The listing builds one solid part. Answer for the finished solid, in the listing's coordinates (mm). A direction names the side the tool comes from. Give positions to 0.01 mm unless a question says otherwise; leave off trailing zeros. Write each loop counter-clockwise with the first axis right and the second up, starting at its lowest first coordinate (ties: lowest second). Pieces come first, ordered by that corner, then holes. Notation, with made-up numbers: (51, 26.25) - (108, 26.25) arc R17 ccw to (108, 48.25) - close; hole circle Ø10 at (-39, 69.25). An arc over 180 degrees is marked (long way). Return JSON: item names as keys, results as strings.
from build123d import *

# Parameters (mm, degrees)
F1_DEPTH = 25.4


with BuildPart() as f1:
    # F0 (on Front) → F1 (new body, symmetric)
    with BuildSketch(Plane.XZ):
        with BuildLine():
            Line((-266.938031, 161.805029), (-266.938031, 123.705029))
            Line((-266.938031, 123.705029), (-228.838031, 123.705029))
            Line((-228.838031, 123.705029), (-204.99998, 176.804662))
            Line((-204.99998, 176.804662), (0, 176.804662))
            Line((0, 176.804662), (28.947621, 122.459758))
            Line((28.947621, 122.459758), (84.925383, 122.459758))
            Line((84.925383, 122.459758), (57.480857, 176.804662))
            Line((57.480857, 176.804662), (98.995887, 157.105953))
            ThreePointArc((98.995887, 157.105953), (109.502053, 158.161564), (114.473462, 167.477085))
            Line((114.473462, 167.477085), (114.473462, 325.248539))
            ThreePointArc((114.473462, 325.248539), (102.023839, 339.250338), (83.320737, 338.137943))
            Line((83.320737, 338.137943), (36.185727, 311.703503))
            Line((36.185727, 311.703503), (-25.528118, 311.703503))
            Line((-25.528118, 311.703503), (-25.528118, 363.759758))
            Line((-25.528118, 363.759758), (-58.593817, 363.759758))
            add(Edge.make_bspline(
                [(-234.475195, 363.759758), (-185.756028, 295.08689), (-104.223274, 299.842954), (-58.593817, 363.759758)],
                knots=[0, 0, 0, 0, 175.881378, 175.881378, 175.881378, 175.881378], degree=3))
            Line((-234.475195, 363.759758), (-266.526538, 363.759758))
            Line((-266.526538, 363.759758), (-266.526538, 311.703503))
            Line((-266.526538, 311.703503), (-180.580374, 233.25789))
            Line((-180.580374, 233.25789), (-236.713991, 233.25789))
            Line((-236.713991, 233.25789), (-266.938031, 161.805029))
        make_face()
        with BuildLine():
            Line((-131.053451, 235.890723), (-73.508778, 286.338449))
            ThreePointArc((-73.508778, 286.338449), (-52.76981, 286.47692), (-49.644388, 265.974343))
            Line((-49.644388, 265.974343), (-90.412526, 201.210762))
            ThreePointArc((-90.412526, 201.210762), (-130.780809, 195.057003), (-131.053451, 235.890723))
        make_face(mode=Mode.SUBTRACT)
        Polygon((30.861216, 235.530361), (16.744013, 214.414855), (-8.655987, 214.414855), (-22.372372, 235.7929), (-8.13638, 256.828502), (17.263144, 256.983855), align=None, mode=Mode.SUBTRACT)
    extrude(amount=F1_DEPTH, both=True)


solid = f1.part
Item 1: A cutting plane is placed at D-D on y = -5. Give the number of separate pieces and of enclosed holes in the cut face, then the cut area to 3 significant figures.
Answer below:
{"separate pieces": "1", "enclosed holes": "2", "area": "54,800 mm²"}
Item 2: The mould has two halves that part along X. Classify faces 4 (the face through (-250, 0, 363.76)), 5 (the face through (-266.938, 0, 143)), 6 (the face through (23.9, -0.36, 225.12)): +X half, -X half, draft (parallel to the pull), parting line (faces both ways), or undercut.
Answer below:
{"face 4": "draft", "face 5": "-X half", "face 6": "undercut"}
Item 3: Flat-ended cylindrical pins translate along their axes: P1, Ø11.5, axis at x = -255.5, y = -12.5, coming from the -Z side (3 decimals); P2, Ø3, axis at x = -47.5, y = 2, coming from the -Z side; P3, Ø1.5, axis at y = -4, z = 337.5, coming from the -X side. Find the tip coordinate at first contact, or state that the pin passes through.
Answer below:
{"P1": "stops at z = 123.705", "P2": "stops at z = 176.8", "P3": "stops at x = -266.53"}
Item 4: For faces 1 (the face through (-15.354, -0.356, 246.163)), 2 (the face through (60.083, -0.356, 325.106)), 3 (the face through (-217.086, -0.356, 149.883)), determine the directions among +Z, -Z, +X, -X, +Y, -Y from which every point of the face is accessible in a straight line to the end or side of a thin tool.
Answer below:
{"face 1": "+Y, -Y", "face 2": "+Z, +Y, -Y", "face 3": "-Z, +Y, -Y"}
Item 5: A cutting plane is placed at C-C on z = 282.5. Determine the outline of the cut face in (x, y), then the cut area to 3 significant figures.
Answer below:
{"outline": "(-234.53, -25.4) - (-77.89, -25.4) - (-77.89, 25.4) - (-234.53, 25.4) - close; (-49.42, -25.4) - (114.47, -25.4) - (114.47, 25.4) - (-49.42, 25.4) - close", "area": "16,300 mm²"}
Item 6: Consider L1, parallel to X at y = -17.5, z = 174; L2, parallel to X at y = 19, z = 245; L3, parallel to Z at x = -195, y = -3. Determine where each line is inside the solid, lowest interval first.
Answer below:
{"L1": "x = -261.78 to -206.26, 1.49 to 58.9, 63.39 to 114.47", "L2": "x = -193.45 to -120.66, -62.85 to -16.14, 24.86 to 114.47", "L3": "z = 176.8 to 233.26, 246.42 to 326.99"}
Item 7: A cutting plane is placed at B-B on z = 223. Determine the outline of the cut face in (x, y), then the cut area to 3 significant figures.
Answer below:
{"outline": "(-241.05, -25.4) - (-139.22, -25.4) - (-139.22, 25.4) - (-241.05, 25.4) - close; (-76.7, -25.4) - (-14.16, -25.4) - (-14.16, 25.4) - (-76.7, 25.4) - close; (22.48, -25.4) - (114.47, -25.4) - (114.47, 25.4) - (22.48, 25.4) - close", "area": "13,000 mm²"}
Item 8: A cutting plane is placed at A-A on x = 24.5. Determine the outline of the cut face in (y, z), then the cut area to 3 significant figures.
Answer below:
{"outline": "(-25.4, 130.81) - (25.4, 130.81) - (25.4, 226.02) - (-25.4, 226.02) - close; (-25.4, 245.57) - (25.4, 245.57) - (25.4, 311.7) - (-25.4, 311.7) - close", "area": "8,200 mm²"}
